Work out the finished part from the listing and answer in its coordinate system (mm). Face numbers are marked on the shaded views. A direction names the side the tool comes from. Coordinates: 2 decimals unless noted, no trailing zeros. Write each loop counter-clockwise with the first axis right and the second up, starting at its lowest first coordinate (ties: lowest second). Pieces come first, ordered by that corner, then holes. Notation, with made-up numbers: (-9.5, -14.5) - (27.5, -14.5) arc R18 cw to (27.5, 19.5) - close; hole circle Ø1 at (63.5, 30). An arc over 180 degrees is marked (long way). Use one line per item in the form item = value. Start each with the question number.
Item 1: Determine the mould class of the marked faces 1, 2 and 3 for opening direction Z: released by +Z, released by -Z, zero draft, split by the parting line, or undercut.
Item 2: A cutting plane is placed at A-A (z = 6.25). Give the number of separate pieces and of enclosed holes in the cut face, then the cut area to 3 significant figures.
Item 3: Given pin 1 (4 mm diameter, centred on y = 16.5, z = 4, fed in from +X); pin 2 (4 mm diameter, centred on y = 20, z = 6.5, fed in from -X); pin 3 (6.5 mm diameter, centred on x = 44.5, z = 7, fed in from -Y); pin 4 (3.5 mm diameter, centred on x = -15.11, z = 6.35, fed in from +Y), each flat-ended and moving along its own axis, determine where each tip first touches the part or whether it passes through.
Item 4: A cutting plane is placed at B-B (y = 22.5). Write down the section's boundary in (x, z).
Item 5: Consider probe 1 along X at (y, z) = (37, 11); probe 2 along X at (y, z) = (24, 1.25); probe 3 along X at (y, z) = (8, 8). Determine where each line is inside the solid, lowest interval first.
Item 6: A cutting plane is placed at D-D (y = 5). Write down the section's boundary in (x, z), then the cut area to 3 significant figures.
Item 7: A cutting plane is placed at C-C (z = 1.25). Write down the section's boundary in (x, y) (3 decimals).
Item 8: For the marked faces 4, 5, 6, 7 and 8, determine the directions among +Z, -Z, +X, -X, +Y, -Y from which every point of the face is accessible in a straight line to the end or side of a thin tool.
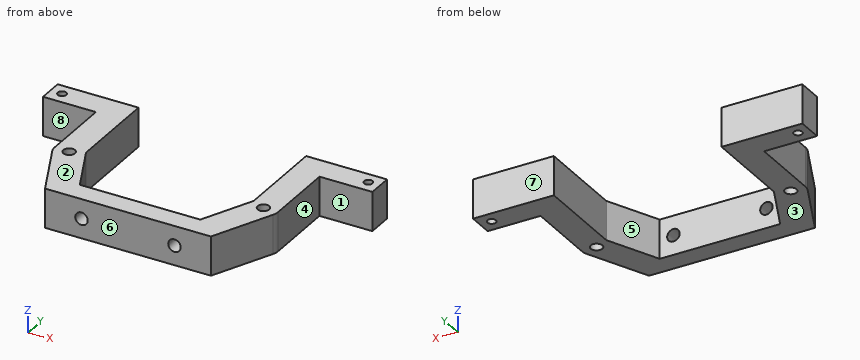
from build123d import *

# Parameters (mm, degrees)
SKETCH1_R      = 1.3716
SKETCH1_R_2    = 1.905
EXTRUDE1_DEPTH = 12.7
SKETCH2_R      = 2.032
EXTRUDE2_DEPTH = 9.652


with BuildPart() as part:
    # Sketch1 → Extrude1 (new body)
    with BuildSketch(Plane.XY):
        with BuildLine():
            Line((-27.225769594, 10.969260914), (-19.564927608, -5.695593273))
            Line((-19.564927608, -5.695593273), (19.564927608, -5.695593273))
            Line((19.564927608, -5.695593273), (27.225769594, 10.969260914))
            Line((27.225769594, 10.969260914), (27.225769594, 40.278404046))
            Line((27.225769594, 40.278404046), (53.492478146, 40.278404046))
            Line((53.492478146, 40.278404046), (53.492478146, 32.09814334))
            Line((53.492478146, 32.09814334), (36.318856593, 32.09814334))
            Line((36.318856593, 32.09814334), (36.318856593, 8.979309022))
            ThreePointArc((36.318856593, 8.979309022), (36.193812026, 7.894938195), (35.825242223, 6.867488665))
            Line((35.825242223, 6.867488665), (26.944030552, -12.452071481))
            Line((26.944030552, -12.452071481), (-26.944030552, -12.452071481))
            Line((-26.944030552, -12.452071481), (-35.825242223, 6.867488665))
            ThreePointArc((-35.825242223, 6.867488665), (-36.193812026, 7.894938195), (-36.318856593, 8.979309022))
            Line((-36.318856593, 8.979309022), (-36.318856593, 32.09814334))
            Line((-36.318856593, 32.09814334), (-53.492478146, 32.09814334))
            Line((-53.492478146, 32.09814334), (-53.492478146, 40.278404046))
            Line((-53.492478146, 40.278404046), (-27.225769594, 40.278404046))
            Line((-27.225769594, 40.278404046), (-27.225769594, 10.969260914))
        make_face()
        with Locations((-49.749305957, 36.28427137)):
            Circle(SKETCH1_R, mode=Mode.SUBTRACT)
        with Locations(Location((49.749305957, 36.28427137, 0), (0, 0, 180))):
            Circle(SKETCH1_R, mode=Mode.SUBTRACT)
        with Locations(Location((31.554570289, 8.979309022, 0), (0, 0, 180))):
            Circle(SKETCH1_R_2, mode=Mode.SUBTRACT)
        with Locations((-31.554570289, 8.979309022)):
            Circle(SKETCH1_R_2, mode=Mode.SUBTRACT)
    extrude(amount=EXTRUDE1_DEPTH)

    # Sketch2 → Extrude2 (cut)
    with BuildSketch(Plane.XZ.offset(12.452071481)):
        with Locations(Location((15.105130103, 6.35, 0), (0, 0, 270))):
            Circle(SKETCH2_R)
        with Locations(Location((-15.105130103, 6.35, 0), (0, 0, 270))):
            Circle(SKETCH2_R)
    extrude(amount=-EXTRUDE2_DEPTH, mode=Mode.SUBTRACT)


solid = part.part
Answer:
q1.face_1 = zero draft
q1.face_2 = released by +Z
q1.face_3 = released by -Z
q2.separate_pieces = 3
q2.enclosed_holes = 4
q2.area = 1,450 mm²
q3.pin_1 = 36.32
q3.pin_2 = -36.32
q3.pin_3 = 32.1
q3.pin_4 = through
q4.outline = (-36.32, 0) - (-27.23, 0) - (-27.23, 12.7) - (-36.32, 12.7) - close; (27.23, 0) - (36.32, 0) - (36.32, 12.7) - (27.23, 12.7) - close
q5.probe_1 = -53.49 to -50.92, -48.58 to -27.23, 27.23 to 48.58, 50.92 to 53.49
q5.probe_2 = -36.32 to -27.23, 27.23 to 36.32
q5.probe_3 = -36.22 to -33.19, -29.92 to -25.86, 25.86 to 29.92, 33.19 to 36.22
q6.outline = (-34.97, 0) - (-24.48, 0) - (-24.48, 12.7) - (-34.97, 12.7) - close; (24.48, 0) - (34.97, 0) - (34.97, 12.7) - (24.48, 12.7) - close
q6.area = 266 mm²
q7.outline = (-53.492, 32.098) - (-36.319, 32.098) - (-36.319, 8.979) arc R4.764 ccw to (-35.825, 6.867) - (-26.944, -12.452) - (26.944, -12.452) - (35.825, 6.867) arc R4.764 ccw to (36.319, 8.979) - (36.319, 32.098) - (53.492, 32.098) - (53.492, 40.278) - (27.226, 40.278) - (27.226, 10.969) - (19.565, -5.696) - (-19.565, -5.696) - (-27.226, 10.969) - (-27.226, 40.278) - (-53.492, 40.278) - close; hole circle Ø2.743 at (-49.749, 36.284); hole circle Ø3.81 at (-31.555, 8.979); hole circle Ø3.81 at (31.555, 8.979); hole circle Ø2.743 at (49.749, 36.284)
q8.face_4 = +Z, -Z, +X, -Y
q8.face_5 = +Z, -Z, +Y
q8.face_6 = +Z, -Z, +X, -X, -Y
q8.face_7 = +Z, -Z, +X, -X, +Y
q8.face_8 = +Z, -Z, -X, -Y
